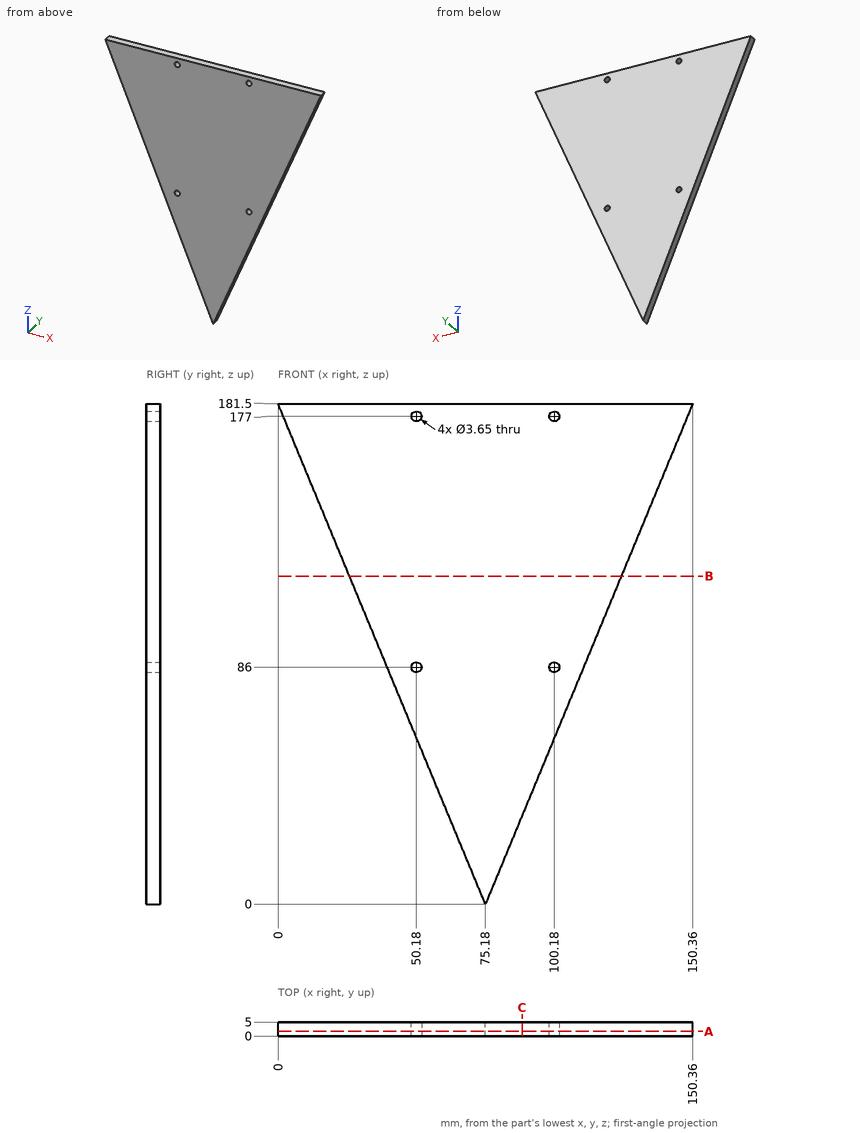
For this review, use the dimensioned drawing (mm, ordinates from the lowest corner) and the shaded views. Round coordinates to 2 decimals unless told otherwise and drop trailing zeros. Write each loop counter-clockwise with the first axis right and the second up, starting at its lowest first coordinate (ties: lowest second). Pieces come first, ordered by that corner, then holes. Notation, with made-up numbers: (-11.75, 52.25) - (18.25, 52.25) arc R20 cw to (18.25, 83.25) - close; hole circle Ø5 at (1, 40). An arc over 180 degrees is marked (long way). Answer as a JSON object with one key per item and string values.
1. To check wall thickness, follow line 1 along X through (y, z) = (1.9, 177) (1 decimal); line 2 along X through (y, z) = (2.15, 86) (1 decimal); line 3 along Z through (x, y) = (49, 3.25) (1 decimal). State the ranges of each line that lie inside material, in increasing order.
Response values:
{"line 1": "x = 1.9 to 48.4, 52 to 98.4, 102 to 148.5", "line 2": "x = 39.6 to 48.4, 52 to 98.4, 102 to 110.8", "line 3": "z = 63.2 to 84.6, 87.4 to 175.6, 178.4 to 181.5"}
2. We need section C-C on x = 88.5. Give the boundary of the cut face in (y, z).
Response values:
{"outline": "(0, 32.16) - (5, 32.16) - (5, 181.5) - (0, 181.5) - close"}
3. We need section A-A on y = 1.7. Count the separate pieces of the cut face and the enclosed holes in it, then the cut area to 3 significant figures.
Response values:
{"separate pieces": "1", "enclosed holes": "4", "area": "13,600 mm2"}
4. For pin 1 Ø3 at (x, z) = (100.18, 86) entering from +Y; pin 2 Ø8 at (x, z) = (93.5, 153) entering from -Y, all flat-tipped, find the tip position at first contact; note any pin that passes through.
Response values:
{"pin 1": "passes through", "pin 2": "stops at y = 0"}
5. We need section B-B on z = 119. Give the boundary of the cut face in (x, y).
Response values:
{"outline": "(25.89, 0) - (124.47, 0) - (124.47, 5) - (25.89, 5) - close"}
